Work out the finished part from the listing and answer in its coordinate system (mm). A direction names the side the tool comes from. Coordinates: 2 decimals unless noted, no trailing zeros. Order: outer loops, then holes, each group sorted by start corner. A loop starts at its lowest first (then second) coordinate and runs counter-clockwise, first axis right, second up. Notation, with made-up numbers: M -15.5,9 L -8.5,9 A27 ccw -8.5,31 Z; hole C 39,84.25 d5. An arc over 180 degrees is marked long. Use a Markdown table: item, result.
from build123d import *

# Parameters (mm, degrees)
BOSS_EXTRUDE1_DEPTH = 50.8
SKETCH7_W           = 228.6
SKETCH7_H           = 152.4
CUT_EXTRUDE5_DEPTH  = 19.05
SKETCH9_R           = 3.3782
CUT_EXTRUDE7_DEPTH  = 27.94
CUT_EXTRUDE8_DEPTH  = 40.64
SKETCH12_W          = 1.27
SKETCH12_H          = 31.75
CUT_EXTRUDE9_DEPTH  = 16.51
CUT_EXTRUDE10_REACH = 33.75
SKETCH13_R          = 3.3782
CUT_EXTRUDE11_DEPTH = 32.75
SKETCH15_R          = 16.002
CUT_EXTRUDE12_DEPTH = 229.6
SKETCH16_W          = 25.4
SKETCH16_H          = 6.35
BOSS_EXTRUDE2_DEPTH = 14.732
SKETCH17_W          = 25.4
SKETCH17_H          = 6.35
BOSS_EXTRUDE3_DEPTH = 14.732
FILLET7_R           = 1.27
FILLET8_R           = 1.27
FILLET9_R           = 1.27
FILLET10_R          = 1.27
CUT_EXTRUDE14_DEPTH = 47.482
FILLET15_R          = 1.27
SKETCH22_R          = 2.286
CUT_EXTRUDE15_DEPTH = 91.697941601


with BuildPart() as part:
    # Sketch2 → Boss-Extrude1 (new body)
    with BuildSketch(Plane.XY):
        with BuildLine():
            Line((215.9, 0), (228.6, 0))
            Line((228.6, 0), (228.6, 101.6))
            Line((228.6, 101.6), (174.752, 152.4))
            Line((174.752, 152.4), (156.972, 152.4))
            ThreePointArc((156.972, 152.4), (143.51, 138.938), (130.048, 152.4))
            Line((130.048, 152.4), (98.552, 152.4))
            ThreePointArc((98.552, 152.4), (85.09, 138.938), (71.628, 152.4))
            Line((71.628, 152.4), (53.848, 152.4))
            Line((53.848, 152.4), (0, 101.6))
            Line((0, 101.6), (0, 0))
            Line((0, 0), (12.7, 0))
            Line((12.7, 0), (215.9, 0))
        make_face()
    extrude(amount=BOSS_EXTRUDE1_DEPTH)

    # Sketch7 → Cut-Extrude5 (cut)
    with BuildSketch(Plane.XY.offset(50.8)):
        with Locations((114.3, 76.2)):
            Rectangle(SKETCH7_W, SKETCH7_H)
    extrude(amount=-CUT_EXTRUDE5_DEPTH, mode=Mode.SUBTRACT)

    # Sketch9 → Cut-Extrude7 (cut)
    with BuildSketch(Plane(origin=(0, 152.4, 0), x_dir=(1, 0, 0), z_dir=(0, 1, 0))):
        with Locations((60.198, -15.875)):
            Circle(SKETCH9_R)
        with Locations((114.3, -15.875)):
            Circle(SKETCH9_R)
        with Locations((168.402, -15.875)):
            Circle(SKETCH9_R)
    extrude(amount=-CUT_EXTRUDE7_DEPTH, mode=Mode.SUBTRACT)

    # Sketch10 → Cut-Extrude8 (cut)
    with BuildSketch(Plane.XY.offset(31.75)):
        Polygon((27.760759157, 101.6), (54.684759157, 127), (173.915240843, 127), (200.839240843, 101.6), align=None)
    extrude(amount=-CUT_EXTRUDE8_DEPTH, mode=Mode.SUBTRACT)

    # Sketch12 → Cut-Extrude9 (cut)
    with BuildSketch(Plane(origin=(0, 152.4, 0), x_dir=(1, 0, 0), z_dir=(0, 1, 0))):
        with Locations((85.725, -15.875)):
            Rectangle(SKETCH12_W, SKETCH12_H)
        with Locations((84.455, -15.875)):
            Rectangle(SKETCH12_W, SKETCH12_H)
        Polygon((143.51, 0), (142.24, 0), (142.24, -31.75), (144.78, -31.75), (144.78, 0), align=None)
    extrude(amount=-CUT_EXTRUDE9_DEPTH, mode=Mode.SUBTRACT)

    # Sketch13 → Cut-Extrude10 (cut, up to next)
    with BuildSketch(Plane.XY.offset(31.75), mode=Mode.PRIVATE) as cut_extrude10_sk1:
        with Locations((45.72, 95.25)):
            Circle(SKETCH13_R)
    cut_extrude10_tool1 = extrude(cut_extrude10_sk1.sketch, amount=-CUT_EXTRUDE10_REACH, mode=Mode.PRIVATE) & part.part
    add(cut_extrude10_tool1.solids().sort_by_distance((45.72, 95.25, 31.75))[0], mode=Mode.SUBTRACT)
    # Sketch13 → Cut-Extrude10 (cut, up to next)
    with BuildSketch(Plane.XY.offset(31.75), mode=Mode.PRIVATE) as cut_extrude10_sk2:
        with Locations((182.88, 95.25)):
            Circle(SKETCH13_R)
    cut_extrude10_tool2 = extrude(cut_extrude10_sk2.sketch, amount=-CUT_EXTRUDE10_REACH, mode=Mode.PRIVATE) & part.part
    add(cut_extrude10_tool2.solids().sort_by_distance((182.88, 95.25, 31.75))[0], mode=Mode.SUBTRACT)

    # Sketch14 → Cut-Extrude11 (cut, through all)
    with BuildSketch(Plane(origin=(0, 0, 0), x_dir=(-1, 0, 0), z_dir=(0, 0, -1))):
        Polygon((-182.88, 59.69), (-228.6, 59.69), (-228.6, 0), (0, 0), (0, 59.69), align=None)
    extrude(amount=-CUT_EXTRUDE11_DEPTH, mode=Mode.SUBTRACT)

    # Sketch15 → Cut-Extrude12 (cut, through all)
    with BuildSketch(Plane(origin=(228.6, 0, 0), x_dir=(0, 0, -1), z_dir=(1, 0, 0))):
        with Locations((-15.875, 59.69)):
            Circle(SKETCH15_R)
    extrude(amount=-CUT_EXTRUDE12_DEPTH, mode=Mode.SUBTRACT)

    # Sketch16 → Boss-Extrude2 (add)
    with BuildSketch(Plane.XY.offset(31.75)):
        with Locations((215.9, 64.877058399)):
            Rectangle(SKETCH16_W, SKETCH16_H)
        with Locations((12.7, 64.877058399)):
            Rectangle(SKETCH16_W, SKETCH16_H)
    extrude(amount=BOSS_EXTRUDE2_DEPTH)

    # Sketch17 → Boss-Extrude3 (add)
    with BuildSketch(Plane(origin=(0, 0, 0), x_dir=(-1, 0, 0), z_dir=(0, 0, -1))):
        with Locations((-215.9, 64.877058399)):
            Rectangle(SKETCH17_W, SKETCH17_H)
        with Locations((-12.7, 64.877058399)):
            Rectangle(SKETCH17_W, SKETCH17_H)
    extrude(amount=BOSS_EXTRUDE3_DEPTH)

    # Fillet7
    fillet7_edges = [part.edges().sort_by_distance(p)[0] for p in [
        (215.9, 68.052058399, 46.482),
    ]]
    fillet(fillet7_edges, radius=FILLET7_R)

    # Fillet8
    fillet8_edges = [part.edges().sort_by_distance(p)[0] for p in [
        (215.9, 68.052058399, -14.732),
    ]]
    fillet(fillet8_edges, radius=FILLET8_R)

    # Fillet9
    fillet9_edges = [part.edges().sort_by_distance(p)[0] for p in [
        (12.7, 68.052058399, -14.732),
    ]]
    fillet(fillet9_edges, radius=FILLET9_R)

    # Fillet10
    fillet10_edges = [part.edges().sort_by_distance(p)[0] for p in [
        (12.7, 68.052058399, 46.482),
    ]]
    fillet(fillet10_edges, radius=FILLET10_R)

    # Sketch20 → Cut-Extrude14 (cut, through all)
    with BuildSketch(Plane.XY.offset(31.75)):
        Polygon((66.04, 61.702058399), (25.4, 61.702058399), (25.4, 78.590265292), (203.2, 78.590265292), (203.2, 61.702058399), (162.56, 61.702058399), align=None)
    extrude(amount=-CUT_EXTRUDE14_DEPTH, mode=Mode.SUBTRACT)

    # Fillet15
    fillet15_edges = [part.edges().sort_by_distance(p)[0] for p in [
        (215.9, 61.702058399, 31.75),
    ]]
    fillet(fillet15_edges, radius=FILLET15_R)

    # Sketch22 → Cut-Extrude15 (cut, through all)
    with BuildSketch(Plane.XZ.offset(-61.702058399)):
        with Locations((12.7, 41.402)):
            Circle(SKETCH22_R)
        with Locations((12.7, -9.652)):
            Circle(SKETCH22_R)
        with Locations((215.9, -9.652)):
            Circle(SKETCH22_R)
        with Locations((215.9, 41.402)):
            Circle(SKETCH22_R)
    extrude(amount=-CUT_EXTRUDE15_DEPTH, mode=Mode.SUBTRACT)


solid = part.part
(1) Which of the six approach directions +Z, -Z, +X, -X, +Y, -Y give full straight-line access (tool end or side, diameter ignored) to faces 1 (the flat face through (216, 61.702, 38)), 2 (the flat face through (113, 78.59, 16)), 3 (the flat face through (65, 152.4, 16)), 4 (the cylindrical face through (133.646, 143.239, 15.653)), 5 (the flat face through (113, 101, 31.75))?
Conclusion:
| item | result |
|---|---|
| face 1 | +Z, -Z, +X, -X, -Y |
| face 2 | +Z, -Z, -Y |
| face 3 | +Z, -Z, +X, -X, +Y |
| face 4 | +Z, -Z, +Y |
| face 5 | +Z, +X, -X, +Y |
(2) A cutting plane is placed at A-A (x = 114.3). Determine the outline of the cut face in (y, z), then the cut area to 3 significant figures.
Conclusion:
| item | result |
|---|---|
| outline | M 78.59,0 L 101.6,0 L 101.6,31.75 L 78.59,31.75 Z; M 127,0 L 152.4,0 L 152.4,12.5 L 127,12.5 Z; M 127,19.25 L 152.4,19.25 L 152.4,31.75 L 127,31.75 Z |
| area | 1,370 mm2 |
(3) A cutting plane is placed at B-B (y = 95.25). Determine the outline of the cut face in (x, z), then the cut area to 3 significant figures.
Conclusion:
| item | result |
|---|---|
| outline | M 0,0 L 42.34,0 L 42.34,31.75 L 0,31.75 Z; M 49.1,0 L 179.5,0 L 179.5,31.75 L 49.1,31.75 Z; M 186.26,0 L 228.6,0 L 228.6,31.75 L 186.26,31.75 Z |
| area | 6,830 mm2 |
(4) A cutting plane is placed at D-D (z = 21.5). Determine the outline of the cut face in (x, y).
Conclusion:
| item | result |
|---|---|
| outline | M 0,74.67 L 25.4,74.67 L 25.4,78.59 L 203.2,78.59 L 203.2,74.67 L 228.6,74.67 L 228.6,101.6 L 174.75,152.4 L 156.97,152.4 A13.46 cw 144.78,139 L 144.78,135.89 L 142.24,135.89 L 142.24,139 A13.46 cw 130.05,152.4 L 98.55,152.4 A13.46 cw 86.36,139 L 86.36,135.89 L 83.82,135.89 L 83.82,139 A13.46 cw 71.63,152.4 L 53.85,152.4 L 0,101.6 Z; hole M 27.76,101.6 L 200.84,101.6 L 173.92,127 L 54.68,127 Z; hole C 45.72,95.25 d6.76; hole C 182.88,95.25 d6.76 |
(5) Determine the mould class of faces 6 (the flat face through (164, 152.4, 16)), 7 (the flat face through (41.03, 114.12, 16.1)), 8 (the cylindrical face through (117.522, 139.878, 14.86)) for opening direction Y: pulls with the +Y half, pulls with the -Y half, needs draft (parallel to the pull), parting line crosses it, or undercut.
Conclusion:
| item | result |
|---|---|
| face 6 | pulls with the +Y half |
| face 7 | undercut |
| face 8 | needs draft |
(6) Straight lines are drawn through the part: L1, parallel to Y at x = 119, z = 5.5; L2, parallel to Z at x = 12, y = 66; L3, parallel to Y at x = 45.5, z = 29. For each, find the intervals that lie inside material, in ascending order.
Conclusion:
| item | result |
|---|---|
| L1 | 78.59 to 101.6, 127 to 152.4 |
| L2 | -14.73 to -11.83, -7.48 to 1.17, 30.58 to 39.23, 43.58 to 46.48 |
| L3 | 78.59 to 91.88, 98.62 to 101.6, 118.34 to 144.52 |
(7) A cutting plane is placed at C-C (x = 32). Determine the outline of the cut face in (y, z), then the cut area to 3 significant figures.
Conclusion:
| item | result |
|---|---|
| outline | M 78.59,0 L 101.6,0 L 101.6,31.75 L 78.59,31.75 Z; M 105.6,0 L 131.79,0 L 131.79,31.75 L 105.6,31.75 Z |
| area | 1,560 mm2 |
(8) Given P1, Ø3, axis at x = 102.5, y = 137.5, coming from the +Z side; P2, Ø2.5, axis at y = 137.5, z = 13.5, coming from the -X side; P3, Ø12, axis at x = 142.5, y = 97.5, coming from the -Z side; P4, Ø4, axis at x = 12.7, z = -9.652, coming from the -Y side, each flat-ended and moving along its own axis, determine where each tip first touches the part or whether it passes through.
Conclusion:
| item | result |
|---|---|
| P1 | z = 31.75 |
| P2 | x = 36.73 |
| P3 | z = 0 |
| P4 | through |
